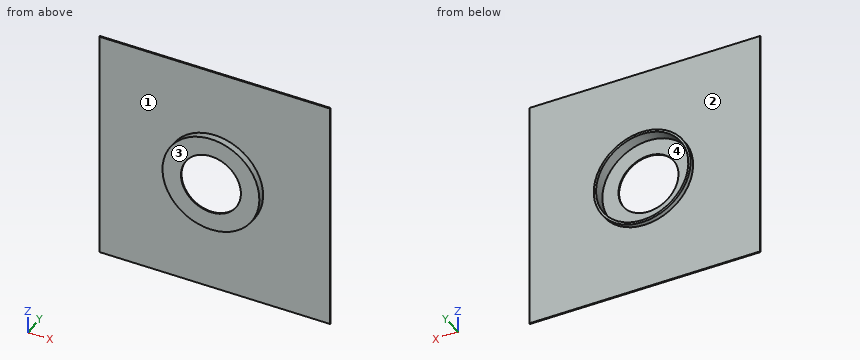
```python
from build123d import *
from build123d.topology import SkipClean

# Parameters (mm, degrees)
SKETCH1_W                = 200
SKETCH1_H                = 200
BOSS_EXTRUDE3_DEPTH      = 1
SKETCH10_R               = 40
CUT_EXTRUDE2_DEPTH       = 1
BOSS_EXTRUDE6_DEPTH      = 5
BOSS_EXTRUDE6_DEPTH_BACK = 5
SKETCH13_R               = 42
SKETCH13_R_2             = 40
SKETCH14_R               = 42
SKETCH14_R_2             = 26
BOSS_EXTRUDE7_DEPTH      = 1


with BuildPart() as part:
    # Sketch1 → Boss-Extrude3 (new body)
    with BuildSketch(Plane(origin=(0, 0, 0), x_dir=(1, 0, 0), z_dir=(0, 1, 0))):
        with Locations((100, -100)):
            Rectangle(SKETCH1_W, SKETCH1_H)
    extrude(amount=BOSS_EXTRUDE3_DEPTH)

    # Sketch10 → Cut-Extrude2 (cut)
    with BuildSketch(Plane(origin=(0, 1, 0), x_dir=(1, 0, 0), z_dir=(0, 1, 0))):
        with Locations(Location((100, -100, 0), (0, 0, 270))):
            Circle(SKETCH10_R)
    extrude(amount=-CUT_EXTRUDE2_DEPTH, mode=Mode.SUBTRACT)

    # Sketch13 → Boss-Extrude6 (add, two sides: drawn at the far end of the back side and taken through both)
    with SkipClean():  # the faces are left unmerged after this step: merging them gives an invalid solid
        with BuildSketch(Plane.XZ.offset(-BOSS_EXTRUDE6_DEPTH_BACK)):
            with Locations(Location((100, 100, 0), (0, 0, 270))):
                Circle(SKETCH13_R)
            with Locations(Location((100, 100, 0), (0, 0, 270))):
                Circle(SKETCH13_R_2, mode=Mode.SUBTRACT)
        extrude(amount=BOSS_EXTRUDE6_DEPTH + BOSS_EXTRUDE6_DEPTH_BACK)

    # Sketch14 → Boss-Extrude7 (add)
    with BuildSketch(Plane.XZ.offset(5)):
        with Locations(Location((100, 100, 0), (0, 0, 270))):
            Circle(SKETCH14_R)
        with Locations(Location((100, 100, 0), (0, 0, 270))):
            Circle(SKETCH14_R_2, mode=Mode.SUBTRACT)
    extrude(amount=BOSS_EXTRUDE7_DEPTH)


solid = part.part
```
The listing builds one solid part. Answer for the finished solid, in the listing's coordinates (mm). Face numbers are marked on the shaded views. A direction names the side the tool comes from. Round coordinates to 2 decimals unless told otherwise and drop trailing zeros. Write each loop counter-clockwise with the first axis right and the second up, starting at its lowest first coordinate (ties: lowest second). Pieces come first, ordered by that corner, then holes. Notation, with made-up numbers: (27, 19.5) -> (39, 19.5) arc R21 ccw to (39, 48.5) -> close; hole circle Ø11 at (-12, 31.5). An arc over 180 degrees is marked (long way). Answer as a JSON object with one key per item and string values. Group by question number.
Q1. Each of these flat-tipped pins is pushed along its axis until it touches: pin 1 Ø24 at (x, z) = (97.5, 97) entering from +Y (1 decimal); pin 2 Ø1 at (y, z) = (-2.5, 110.5) entering from -X; pin 3 Ø1 at (x, z) = (56.5, 28.5) entering from +Y. Where does it stop, or does it pass through?
Q2. Which of the six approach directions +Z, -Z, +X, -X, +Y, -Y give full straight-line access (tool end or side, diameter ignored) to the marked faces 1 and 2?
Q3. Section A-A (z = 100) is taken. Write down the section's boundary in (x, y), plus the area to 3 significant figures.
Q4. Determine the mould class of the marked faces 3 and 4 for opening direction Z: pulls with the +Z half, pulls with the -Z half, needs draft (parallel to the pull), parting line crosses it, or undercut.
Q5. Section C-C (z = 135) is taken. Write down the section's boundary in (x, y).
Q6. Straight lines are drawn through the part: line 1 along X through (y, z) = (-5.5, 98.5); line 2 along Y through (x, z) = (118, 59); line 3 along X through (y, z) = (-2.25, 100). For each, find the intervals that lie inside material, in ascending order.
Q7. Section D-D (x = 38.5) is taken. Write down the section's boundary in (y, z), plus the area to 3 significant figures.
Q8. Section B-B (x = 100) is taken. Write down the section's boundary in (y, z).
Check values:
{
 "1": {"pin 1": "through", "pin 2": "x = 59.21", "pin 3": "y = 1"},
 "2": {"face 1": "-Y", "face 2": "+Y"},
 "3": {"outline": "(0, 0) -> (58, 0) -> (58, -6) -> (74, -6) -> (74, -5) -> (60, -5) -> (60, 5) -> (58, 5) -> (58, 1) -> (0, 1) -> close; (126, -6) -> (142, -6) -> (142, 0) -> (200, 0) -> (200, 1) -> (142, 1) -> (142, 5) -> (140, 5) -> (140, -5) -> (126, -5) -> close", "area": "188 mm^2"},
 "4": {"face 3": "needs draft", "face 4": "undercut"},
 "5": {"outline": "(0, 0) -> (76.78, 0) -> (76.78, -6) -> (123.22, -6) -> (123.22, 0) -> (200, 0) -> (200, 1) -> (123.22, 1) -> (123.22, 5) -> (119.36, 5) -> (119.36, -5) -> (80.64, -5) -> (80.64, 5) -> (76.78, 5) -> (76.78, 1) -> (0, 1) -> close"},
 "6": {"line 1": "58.03 to 74.04, 125.96 to 141.97", "line 2": "0 to 1", "line 3": "58 to 60, 140 to 142"},
 "7": {"outline": "(0, 0) -> (1, 0) -> (1, 200) -> (0, 200) -> close", "area": "200 mm^2"},
 "8": {"outline": "(-6, 58) -> (0, 58) -> (0, 0) -> (1, 0) -> (1, 58) -> (5, 58) -> (5, 60) -> (-5, 60) -> (-5, 74) -> (-6, 74) -> close; (-6, 126) -> (-5, 126) -> (-5, 140) -> (5, 140) -> (5, 142) -> (1, 142) -> (1, 200) -> (0, 200) -> (0, 142) -> (-6, 142) -> close"}
}
